Here's how the part is built. I have some questions about the finished solid (model axes, mm). A direction names the side the tool comes from. Round coordinates to 2 decimals unless told otherwise and drop trailing zeros. Write each loop counter-clockwise with the first axis right and the second up, starting at its lowest first coordinate (ties: lowest second). Pieces come first, ordered by that corner, then holes. Notation, with made-up numbers: (41, 50.25) -> (63, 50.25) arc R5 ccw to (63, 56.25) -> close; hole circle Ø11 at (68, 32.5). An arc over 180 degrees is marked (long way). Answer as CSV lines item,"result".
```python
from build123d import *

# Parameters (mm, degrees)
F0_W     = 550
F0_H     = 50
F0_H_2   = 420
F0_W_2   = 120
F0_H_3   = 120
F1_DEPTH = 18


with BuildPart() as f1:
    # F0 (on Front) → F1 (new body)
    with BuildSketch(Plane.XZ):
        with Locations((0, -235)):
            Rectangle(F0_W, F0_H)
        Rectangle(F0_W, F0_H_2)
        with Locations((175, 110)):
            Rectangle(F0_W_2, F0_H_3, mode=Mode.SUBTRACT)
        with Locations((0, 235)):
            Rectangle(F0_W, F0_H)
    extrude(amount=F1_DEPTH)


solid = f1.part
```
1. Suppose I cut it at C-C on x = 203.5. Please give me the cut outline in (y, z).
Numbers:
outline,"(-18, -260) -> (0, -260) -> (0, 50) -> (-18, 50) -> close; (-18, 170) -> (0, 170) -> (0, 260) -> (-18, 260) -> close"
2. Suppose I cut it at B-B on z = 57.5. Please give me the cut outline in (x, y), and give its area (3 significant figures).
Numbers:
outline,"(-275, -18) -> (115, -18) -> (115, 0) -> (-275, 0) -> close; (235, -18) -> (275, -18) -> (275, 0) -> (235, 0) -> close"
area,"7,740 mm^2"
3. If I drill on line 1 (Z direction, x = 234, y = -4.5); line 2 (X direction, y = -12.5, z = 165), over which ranges is the centre line in solid material (lowest first)?
Numbers:
line 1,"z = -260 to 50, 170 to 260"
line 2,"x = -275 to 115, 235 to 275"
4. Suppose I cut it at A-A on y = -13.25. Please give me the cut outline in (x, z).
Numbers:
outline,"(-275, -260) -> (275, -260) -> (275, 260) -> (-275, 260) -> close; hole (115, 50) -> (235, 50) -> (235, 170) -> (115, 170) -> close"
5. If we mould it in two halves opening along X, with no side actions, what happens to faces 3 (the face through (-275, -9, 4)), 4 (the face through (-4, -9, -260)), 5 (the face through (115, -9, 109))? For each: released by +X, released by -X, zero draft, split by the parting line, or undercut.
Numbers:
face 3,"released by -X"
face 4,"zero draft"
face 5,"undercut"
6. On a 3-axis mill with a long thin cutter (end or side, diameter ignored), from which of +Z, -Z, +X, -X, +Y, -Y can I reach the whole of each face in a straight line? I mean faces 1 (the face through (-4, -9, 260)), 2 (the face through (174, -9, 50)). Say none if no direction works.
Numbers:
face 1,"+Z, +X, -X, +Y, -Y"
face 2,"+Y, -Y"
7. For pin 1 Ø1.5 at (x, z) = (5.5, 90.5) entering from +Y, with a flat end and sliding along its axis, tell me the tip position at first contact or that it passes through.
Numbers:
pin 1,"stops at y = 0"
